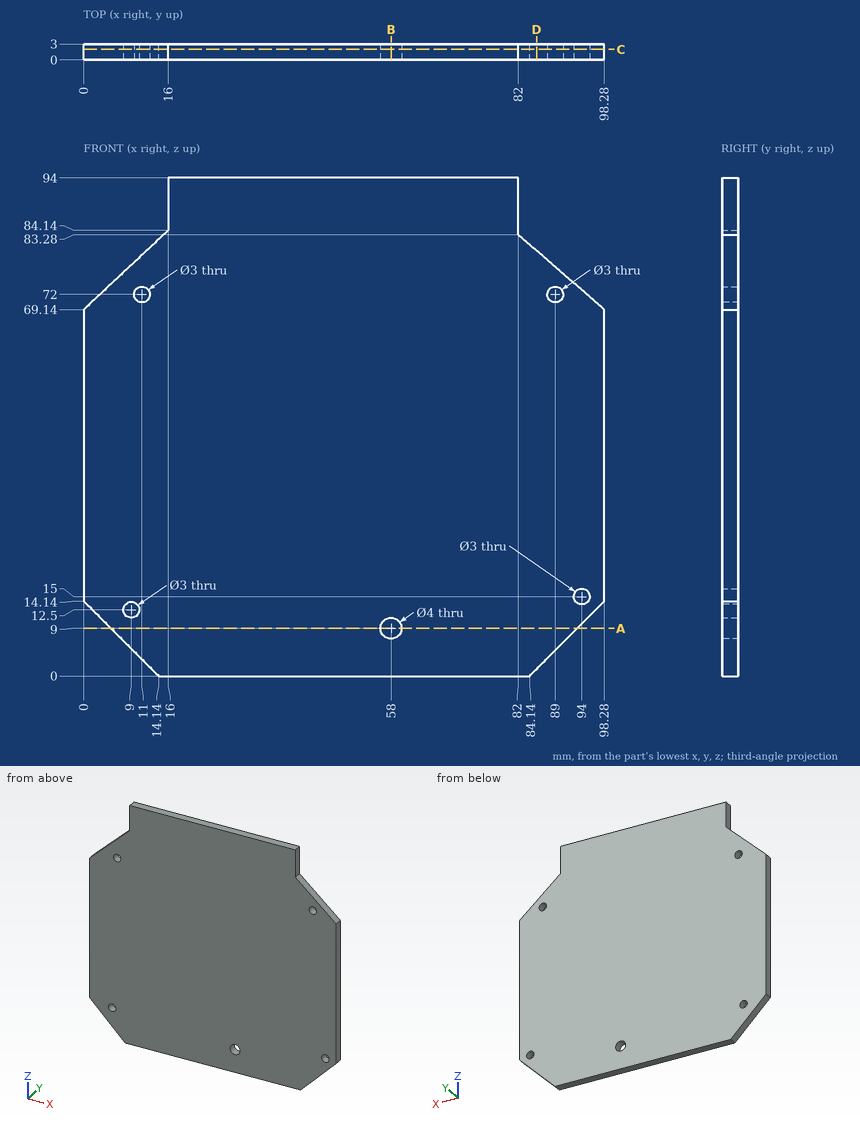
Study the drawing (mm; zero at the part's minimum x, y, z) and answer. Round coordinates to 2 decimals unless told otherwise and drop trailing zeros. Write each loop counter-clockwise with the first axis right and the second up, starting at its lowest first coordinate (ties: lowest second). Pieces come first, ordered by that corner, then holes. Notation, with made-up numbers: (24.25, 19) - (35.25, 19) arc R26 ccw to (35.25, 58) - close; hole circle Ø6 at (9, 39). An arc over 180 degrees is marked (long way). Use CSV: the item, a comma, the result in double quotes.
Q1. Each of these flat-tipped pins is pushed along its axis until it touches: pin 1 Ø3.5 at (x, z) = (58, 9) entering from +Y; pin 2 Ø0.9 at (y, z) = (2, 89) entering from -X. Where does it stop, or does it pass through?
Values:
pin 1,"passes through"
pin 2,"stops at x = 16"
Q2. Find section C-C, the plane y = 2. Write down the section's boundary in (x, z), then the cut area to 3 significant figures.
Values:
outline,"(0, 14.14) - (14.14, 0) - (84.14, 0) - (98.28, 14.14) - (98.28, 69.14) - (82, 83.28) - (82, 94) - (16, 94) - (16, 84.14) - (0, 69.14) - close; hole circle Ø3 at (9, 12.5); hole circle Ø3 at (11, 72); hole circle Ø4 at (58, 9); hole circle Ø3 at (89, 72); hole circle Ø3 at (94, 15)"
area,"8,430 mm²"
Q3. Find section A-A, the plane z = 9. Write down the section's boundary in (x, y), then the cut area to 3 significant figures.
Values:
outline,"(5.14, 0) - (56, 0) - (56, 3) - (5.14, 3) - close; (60, 0) - (93.14, 0) - (93.14, 3) - (60, 3) - close"
area,"252 mm²"
Q4. Straight lines are drawn through the part: line 1 along X through (y, z) = (1.6, 72); line 2 along Z through (x, y) = (89, 2.3); line 3 along Z through (x, y) = (94, 1.5). For each, find the intervals that lie inside material, in ascending order.
Values:
line 1,"x = 3.05 to 9.5, 12.5 to 87.5, 90.5 to 94.99"
line 2,"z = 4.86 to 70.5, 73.5 to 77.2"
line 3,"z = 9.86 to 13.5, 16.5 to 72.86"
Q5. Find section B-B, the plane x = 58. Write down the section's boundary in (y, z), then the cut area to 3 significant figures.
Values:
outline,"(0, 0) - (3, 0) - (3, 7) - (0, 7) - close; (0, 11) - (3, 11) - (3, 94) - (0, 94) - close"
area,"270 mm²"
Q6. Find section D-D, the plane x = 85.5. Write down the section's boundary in (y, z).
Values:
outline,"(0, 1.36) - (3, 1.36) - (3, 80.24) - (0, 80.24) - close"
